Work out the finished part from the listing and answer in its coordinate system (mm). A direction names the side the tool comes from. Coordinates: 2 decimals unless noted, no trailing zeros. Write each loop counter-clockwise with the first axis right and the second up, starting at its lowest first coordinate (ties: lowest second). Pieces come first, ordered by that corner, then holes. Notation, with made-up numbers: (-17, 75.25) -> (-5, 75.25) arc R7 ccw to (-5, 82.25) -> close; hole circle Ø5 at (41.25, -7.75). An arc over 180 degrees is marked (long way). Write each question's results on one line, items separated by ' | '. Start each with the question number.
from build123d import *

# Parameters (mm, degrees)
MODEL_R           = 1.4
MODEL_R_2         = 1
BRIDA_BASE1_DEPTH = 1


# Sheet-metal steps are written as plain solids
with BuildPart() as part:
    # Model → Brida base1 (new body)
    with BuildSketch(Plane.XY):
        with BuildLine():
            Line((50.207437074, -7.391699149), (48.298711017, 1.436394934))
            Line((48.298711017, 1.436394934), (47.876387864, 2.792489658))
            ThreePointArc((47.876387864, 2.792489658), (47.852286656, 3.315621633), (48.087445951, 3.783540469))
            Line((48.087445951, 3.783540469), (51.948138549, 8.171489457))
            ThreePointArc((51.948138549, 8.171489457), (52.139383389, 8.489686819), (52.2059904, 8.854909567))
            Line((52.2059904, 8.854909567), (52.2059904, 33.853262145))
            ThreePointArc((52.2059904, 33.853262145), (51.2059904, 34.853262145), (50.2059904, 33.853262145))
            Line((50.2059904, 33.853262145), (50.2059904, 13.851710132))
            ThreePointArc((50.2059904, 13.851710132), (49.912550656, 13.14560465), (49.205991599, 12.853258732))
            Line((49.205991599, 12.853258732), (47.205989201, 12.853258732))
            ThreePointArc((47.205989201, 12.853258732), (46.499430144, 13.14560465), (46.2059904, 13.851710132))
            Line((46.2059904, 13.851710132), (46.2059904, 33.853262145))
            ThreePointArc((46.2059904, 33.853262145), (45.2059904, 34.853262145), (44.2059904, 33.853262145))
            Line((44.2059904, 33.853262145), (44.2059904, 13.853262145))
            ThreePointArc((44.2059904, 13.853262145), (43.913097181, 13.146155364), (43.2059904, 12.853262145))
            Line((43.2059904, 12.853262145), (41.261682565, 12.853262145))
            ThreePointArc((41.261682565, 12.853262145), (40.55729517, 13.146045419), (40.26429965, 13.850344556))
            Line((40.26429965, 13.850344556), (40.2059904, 33.859090521))
            ThreePointArc((40.2059904, 33.859090521), (39.203084692, 34.853266391), (38.2059904, 33.853262145))
            Line((38.2059904, 33.853262145), (38.278848795, 8.854909567))
            ThreePointArc((38.278848795, 8.854909567), (38.330209967, 8.450786945), (38.53359758, 8.097818756))
            Line((38.53359758, 8.097818756), (42.324534849, 3.783540469))
            ThreePointArc((42.324534849, 3.783540469), (42.559377318, 3.315539648), (42.534995737, 2.792489658))
            Line((42.534995737, 2.792489658), (42.111984195, 1.436609508))
            Line((42.111984195, 1.436609508), (40.20743717, -7.393077864))
            Line((40.20743717, -7.393077864), (40.208815885, -17.393077769))
            ThreePointArc((40.208815885, -17.393077769), (45.208815932, -22.393077817), (50.20881598, -17.393077769))
            Line((50.20881598, -17.393077769), (50.207437074, -7.391699149))
        make_face()
        with Locations((45.208815932, -17.393077769)):
            Circle(MODEL_R, mode=Mode.SUBTRACT)
        with Locations((45.208815932, -4.893077769)):
            Circle(MODEL_R_2, mode=Mode.SUBTRACT)
    extrude(amount=-BRIDA_BASE1_DEPTH)


solid = part.part
1. Find section C-C on z = -0.75. Give the number of separate pieces and of enclosed holes in the cut face, and give its area (3 significant figures).
2. For faces 1 (the face through (41.173, -2.916, -0.493)), 2 (the face through (46.206, 23.7, -0.5)), 3 (the face through (49.266, -3.039, -0.493)), determine the directions among +Z, -Z, +X, -X, +Y, -Y from which every point of the face is accessible in a straight line to the end or side of a thin tool.
3. Find the intervals of material crossed by L1, parallel to X at y = -17.5, z = -0.55; L2, parallel to Y at x = 45, z = -0.45; L3, parallel to Y at x = 44.5, z = -0.3, in increasing order.
4. Given pin 1 Ø2 at (x, y) = (45.21, -17.39) entering from +Z; pin 2 Ø0.5 at (y, z) = (-13.5, -0.5) entering from -X, each flat-ended and moving along its own axis, determine where each tip first touches the part or whether it passes through.
5. Find section B-B on x = 45. Give the vertices of the cut face in (y, z).
6. Find section A-A on y = 25.5. Give the vertices of the cut face in (x, z), and give its area (3 significant figures).
7. Find section D-D on y = 6. Give the vertices of the cut face in (x, z), and give its area (3 significant figures).
8. Determine the mould class of faces 4 (the face through (45, 0, 0)), 5 (the face through (45.228, 34.853, -0.493)), 6 (the face through (47.85, 3.31, -0.49)) for opening direction Y: pulls with the +Y half, pulls with the -Y half, needs draft (parallel to the pull), parting line crosses it, or undercut.
Ans:
1) separate pieces: 1 | enclosed holes: 2 | area: 453 mm²
2) face 1: +Z, -Z, -X | face 2: +Z, -Z, +Y | face 3: +Z, -Z, +X
3) L1: x = 40.21 to 43.81, 46.6 to 50.21 | L2: y = -22.39 to -18.78, -16.01 to -5.87, -3.92 to 34.83 | L3: y = -22.34 to -18.6, -16.19 to -5.6, -4.19 to 34.56
4) pin 1: passes through | pin 2: stops at x = 40.21
5) outline: (-22.39, -1) -> (-18.78, -1) -> (-18.78, 0) -> (-22.39, 0) -> close; (-16.01, -1) -> (-5.87, -1) -> (-5.87, 0) -> (-16.01, 0) -> close; (-3.92, -1) -> (34.83, -1) -> (34.83, 0) -> (-3.92, 0) -> close
6) outline: (38.23, -1) -> (40.23, -1) -> (40.23, 0) -> (38.23, 0) -> close; (44.21, -1) -> (46.21, -1) -> (46.21, 0) -> (44.21, 0) -> close; (50.21, -1) -> (52.21, -1) -> (52.21, 0) -> (50.21, 0) -> close | area: 6.00 mm²
7) outline: (40.38, -1) -> (50.04, -1) -> (50.04, 0) -> (40.38, 0) -> close | area: 9.66 mm²
8) face 4: needs draft | face 5: pulls with the +Y half | face 6: undercut
